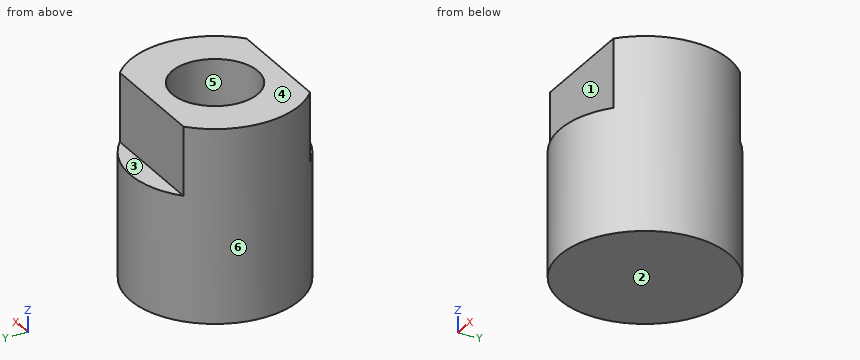
from build123d import *

# Parameters (mm, degrees)
F0_R     = 3.95
F1_DEPTH = 9
F3_DEPTH = 3.2
F4_R     = 2
F5_DEPTH = 8


with BuildPart() as f1:
    # F0 (on Top) → F1 (new body)
    with BuildSketch(Plane.XY):
        Circle(F0_R)
    extrude(amount=F1_DEPTH)

    # F2 (on face) → F3 (cut)
    with BuildSketch(Plane.XY.offset(9)):
        with BuildLine():
            Line((2.626785, -2.95), (-2.626785, -2.95))
            ThreePointArc((-2.626785, -2.95), (0, -3.95), (2.626785, -2.95))
        make_face()
        with BuildLine():
            ThreePointArc((2.626785, 2.95), (0, 3.95), (-2.626785, 2.95))
            Line((-2.626785, 2.95), (2.626785, 2.95))
        make_face()
    extrude(amount=-F3_DEPTH, mode=Mode.SUBTRACT)

    # F4 (on face) → F5 (cut)
    with BuildSketch(Plane.XY.offset(9)):
        Circle(F4_R)
    extrude(amount=-F5_DEPTH, mode=Mode.SUBTRACT)


solid = f1.part
Can you work these out from the model? Positions are in its coordinate system, mm. Face numbers are marked on the shaded views. A direction names the side the tool comes from. Give positions to 0.01 mm unless a question says otherwise; leave off trailing zeros. Loops run counter-clockwise (first coordinate to the right, second up) from the corner with the lowest first, then second, coordinate; pieces in that order, holes last. Notation, with made-up numbers: (86, 43) - (95, 43) arc R37 ccw to (95, 82) - close; hole circle Ø7 at (6.25, 65.5). An arc over 180 degrees is marked (long way). One line per item, written item: value.
(1) If we section it at C-C, the plane z = 3: List the corners of the cut face in (x, y) for me.
Verdict:
outline: circle Ø7.9 at (0, 0); hole circle Ø4 at (0, 0)
(2) On a 3-axis mill with a long thin cutter (end or side, diameter ignored), from which of +Z, -Z, +X, -X, +Y, -Y can I reach the whole of each face in a straight line? I mean the marked faces 1, 2 and 3. Say none if no direction works.
Verdict:
face 1: +Z, +X, -X, -Y
face 2: -Z, +X, -X, +Y, -Y
face 3: +Z, +X, -X, +Y
(3) I need wall thicknesses on line 1 along Y through (x, z) = (0, 5); line 2 along Y through (x, z) = (0, 6.75); line 3 along Z through (x, y) = (0, 0.25). Which ranges of each line are inside material? Lowest first, please.
Verdict:
line 1: -3.95 to -2, 2 to 3.95
line 2: -2.95 to -2, 2 to 2.95
line 3: 0 to 1
(4) If we section it at A-A, the plane y = 0: List the corners of the cut face in (x, z) for me, plus the area to 3 significant figures.
Verdict:
outline: (-3.95, 0) - (3.95, 0) - (3.95, 9) - (2, 9) - (2, 1) - (-2, 1) - (-2, 9) - (-3.95, 9) - close
area: 39.1 mm^2
(5) If we section it at B-B, the plane x = 0: List the corners of the cut face in (y, z) for me, plus the area to 3 significant figures.
Verdict:
outline: (-3.95, 0) - (3.95, 0) - (3.95, 5.8) - (2.95, 5.8) - (2.95, 9) - (2, 9) - (2, 1) - (-2, 1) - (-2, 9) - (-2.95, 9) - (-2.95, 5.8) - (-3.95, 5.8) - close
area: 32.7 mm^2
(6) If we mould it in two halves opening along Y, with no side actions, what happens to the marked faces 4, 5 and 6? For each: released by +Y, released by -Y, zero draft, split by the parting line, or undercut.
Verdict:
face 4: zero draft
face 5: undercut
face 6: split by the parting line
(7) I'm going to push flat-ended pins straight in: pin 1 (2 mm diameter, centred on x = -0.5, y = -0.5, fed in from +Z); pin 2 (1 mm diameter, centred on x = -1, z = 7.5, fed in from -Y); pin 3 (4 mm diameter, centred on x = 1.5, y = 1.5, fed in from -Z); pin 4 (2.5 mm diameter, centred on x = -1, z = 8, fed in from +Y). Where does each tip first touch, or does it pass through?
Verdict:
pin 1: z = 1
pin 2: y = -2.95
pin 3: z = 0
pin 4: y = 2.95
(8) If we section it at D-D, the plane x = -2.5: List the corners of the cut face in (y, z) for me.
Verdict:
outline: (-3.06, 0) - (3.06, 0) - (3.06, 5.8) - (2.95, 5.8) - (2.95, 9) - (-2.95, 9) - (-2.95, 5.8) - (-3.06, 5.8) - close
